For this review, take the finished solid that the model builds, in its own axes (mm). A direction names the side the tool comes from. Coordinates: 2 decimals unless noted, no trailing zeros. Write each loop counter-clockwise with the first axis right and the second up, starting at its lowest first coordinate (ties: lowest second). Pieces come first, ordered by that corner, then holes.
1) We need section A-A on y = 355.6. Write out the cut boundary in (x, z) (1 decimal), then the cut area to 3 significant figures.
2) To check wall thickness, follow line 1 along X through (y, z) = (186.5, -28.5) (3 decimals); line 2 along Y through (x, z) = (-23.1, -25.4); line 3 along Z through (x, y) = (-1.05, 12.7). State the ranges of each line that lie inside material, in increasing order.
3) Mouldability with a two-part tool opening along X and no side actions: class faces 1 (the face through (0, 188, -26)), 2 (the face through (-23.79, 207.814, -6.682)), 3 (the face through (-3.175, 188, -26)) as pulls with the +X half, pulls with the -X half, needs draft (parallel to the pull), parting line crosses it, or undercut.
4) We need section C-C on y = 99.5. Write out the cut boundary in (x, z) (3 decimals).
5) Insertion check: P1, Ø9, axis at y = 247.14, z = -43.36, coming from the +X side. The pin has a flat end and moves straight along its axis. Give the tip position at first contact, or say it passes through.
6) For faces 4 (the face through (-13, 188, -3.175)), 5 (the face through (-2, 381, -27)), list the 3-axis set-ups (+Z, -Z, +X, -X, +Y, -Y) from which the entire face can be reached by the end or side of a thin tool; tool diameter is ignored.
7) We need section B-B on x = -10. Write out the cut boundary in (y, z) (3 decimals).
Autodesk Inventor part; units mm, degrees
ref_plane "YZ Plane" through (0, 0, 0) normal (1, 0, 0) x (0, 1, 0)
ref_plane "XZ Plane" through (0, 0, 0) normal (0, 1, 0) x (-1, 0, 0)
ref_plane "XY Plane" through (0, 0, 0) normal (0, 0, 1) x (1, 0, 0)
sketch "Sketch1" plane through (0, 0, 0) normal (0, 1, 0) x (-1, 0, 0)
  line L0 (0, 0) -> (25.4, 0)
  line L1 (25.4, 0) -> (25.4, -50.8)
  line L2 (25.4, -50.8) -> (0, -50.8)
  line L3 (0, -50.8) -> (0, 0)
  dimension "d0" = 25.4
  dimension "d1" = 50.8
extrude "Extrusion1" add sketch "Sketch1" along normal blind 381
shell "Shell1" thickness 3.175 removed faces 2 at (-8.4667, 0, -33.8667) at (-8.4667, 381, -33.8667)
sketch "Sketch2" plane through (0, 0, 0) normal (1, 0, 0) x (0, 0, -1)
  line L0 (0, 0) -> (0, 381)
  line L1 (0, 12.7) -> (50.8, 12.7)
  line L2 (50.8, 0) -> (50.8, 381)
  circle A0 centre (25.4, 12.7) radius 2.0701
  circle A1 centre (38.1, 12.7) radius 2.0701
  circle A2 centre (12.7, 12.7) radius 2.0701
  line L3 (0, 0) -> (50.8, 0)
  line L4 (3.175, 381) -> (47.625, 381)
  line L5 (25.4, 381) -> (25.4, 355.6)
  circle A3 centre (25.4, 355.6) radius 14.2875
  line L6 (25.4, 355.6) -> (25.4, 229.1842)
  circle A4 centre (25.4, 229.1842) radius 14.2875
  circle A5 centre (25.4, 229.1842) radius 25.4 construction
  line L7 (25.4, 229.1842) -> (43.3605, 247.1447) construction
  line L8 (25.4, 229.1842) -> (50.8, 229.1842) construction
  line L9 (25.4, 229.1842) -> (43.3605, 211.2237) construction
  line L10 (25.4, 229.1842) -> (7.4395, 211.2237) construction
  line L11 (25.4, 229.1842) -> (7.4395, 247.1447) construction
  circle A6 centre (7.4395, 247.1447) radius 3.4925
  circle A7 centre (43.3605, 247.1447) radius 3.4925
  circle A8 centre (43.3605, 211.2237) radius 3.4925
  circle A9 centre (7.4395, 211.2237) radius 3.4925
  dimension "d5" = 4.1402
  dimension "d8" = 12.7
  dimension "d15" = 12.7
  dimension "d22" = 12.7
  dimension "d23" = 25.4
  dimension "d24" = 28.575
  dimension "d25" = 28.575
  dimension "d26" = 126.4158
  dimension "d27" = 50.8
  dimension "d28" = 45
  dimension "d29" = 6.985
  dimension "d30" = 6.985
  dimension "d31" = 6.985
  dimension "d32" = 6.985
extrude "Extrusion2" cut sketch "Sketch2" against normal through all contours A2 L1 | L1 A2 | A1 L1 | L1 A1 | A0 L1 | L1 A0 | A3 L6 L5 | A4 | L5 L6 A3 | A6 | A7 | A8 | A9
properties part number "Arm Mount"
Result:
1. outline: (-25.4, -50.8) - (0, -50.8) - (0, -39.7) - (-3.2, -39.7) - (-3.2, -47.6) - (-22.2, -47.6) - (-22.2, -39.7) - (-25.4, -39.7) - close; (-25.4, -11.1) - (-22.2, -11.1) - (-22.2, -3.2) - (-3.2, -3.2) - (-3.2, -11.1) - (0, -11.1) - (0, 0) - (-25.4, 0) - close
1. area: 262 mm2
2. line 1: x = -25.4 to -22.225, -3.175 to 0
2. line 2: y = 0 to 10.63, 14.77 to 214.9, 243.47 to 341.31, 369.89 to 381
2. line 3: z = -50.8 to -40.17, -36.03 to -27.47, -23.33 to -14.77, -10.63 to 0
3. face 1: pulls with the +X half
3. face 2: needs draft
3. face 3: undercut
4. outline: (-25.4, -50.8) - (0, -50.8) - (0, 0) - (-25.4, 0) - close; hole (-22.225, -47.625) - (-3.175, -47.625) - (-3.175, -3.175) - (-22.225, -3.175) - close
5. P1: stops at x = 0
6. face 4: +Y, -Y
6. face 5: +Z, -Z, +X, -X, +Y
7. outline: (0, -50.8) - (381, -50.8) - (381, -47.625) - (0, -47.625) - close; (0, -3.175) - (381, -3.175) - (381, 0) - (0, 0) - close
